```python
from build123d import *
from build123d import SkipClean  # not in build123d's __all__

# Parameters (mm, degrees)
F0_R        = 4.7625
F1_DEPTH    = 1.5875
F3_DEPTH    = 4.7625
F4_T1_DEPTH = 17.0592221242


# Not quite as in the source:
# - a fillet or chamfer that OpenCascade refuses, or shapes differently, is made with other operations: its cross-section is extruded or revolved along the edge and cut away or added


with BuildPart() as f1:
    # F0 (on Top) → F1 (new body)
    with BuildSketch(Plane.XY):
        with BuildLine():
            Line((-10.31875, 4.7625), (-10.31875, 0))
            ThreePointArc((-10.31875, 0), (0, -10.31875), (10.31875, 0))
            Line((10.31875, 0), (10.31875, 4.7625))
            ThreePointArc((10.31875, 4.7625), (0, 15.08125), (-10.31875, 4.7625))
        make_face()
        with Locations((0, -0.79375)):
            Circle(F0_R, mode=Mode.SUBTRACT)
    extrude(amount=F1_DEPTH)

    # F2 (on face) → F3 (join)
    with BuildSketch(Plane.XY.offset(1.5875)):
        with BuildLine():
            ThreePointArc((-4.7625, -0.79375), (0, 3.96875), (4.7625, -0.79375))
            Line((4.7625, -0.79375), (4.7625, 5.55625))
            ThreePointArc((4.7625, 5.55625), (0, 10.31875), (-4.7625, 5.55625))
            Line((-4.7625, 5.55625), (-4.7625, -0.79375))
        make_face()
    with SkipClean():  # cleaning this boolean's faces spoils the solid; the shape is the same uncleaned
        extrude(amount=F3_DEPTH)

    # F4: fillet of radius 1.27 on 2 edges, made by hand

    # F4_s2 → F4_t1 (cut)
    with BuildSketch(Plane.XY.offset(1.5875)):
        with BuildLine():
            ThreePointArc((4.7625, 4.1249388497), (4.075215964, 2.9965142376), (2.7572368421, 3.0894254076))
            ThreePointArc((2.7572368421, 3.0894254076), (4.2315922955, 1.3914348651), (4.7625, -0.79375))
            Line((4.7625, -0.79375), (4.7625, 4.1249388497))
        make_face()
        with BuildLine():
            ThreePointArc((-4.7625, 4.1249388497), (-4.075215964, 2.9965142376), (-2.7572368421, 3.0894254076))
            ThreePointArc((-2.7572368421, 3.0894254076), (-4.2315922955, 1.3914348651), (-4.7625, -0.79375))
            Line((-4.7625, -0.79375), (-4.7625, 4.1249388497))
        make_face()
    extrude(amount=F4_T1_DEPTH, mode=Mode.SUBTRACT)


solid = f1.part
```
Source: CAD feature listing. Evaluate the final solid. Frame: model axes, mm. A direction names the side the tool comes from. Give positions to 0.01 mm unless a question says otherwise; leave off trailing zeros. Loops run counter-clockwise (first coordinate to the right, second up) from the corner with the lowest first, then second, coordinate; pieces in that order, holes last. Notation, with made-up numbers: (29, 43) -> (44, 43) arc R22 ccw to (44, 68) -> close; hole circle Ø8 at (70.25, 78). An arc over 180 degrees is marked (long way). Put each result on its own line as item: value. Start each with the question number.
1) Cut plane A-A (x = 0). Return loops of the section in (y, z).
2) Contact query for flat-ended pins moving along their axis: P1, Ø1.5, axis at x = 4, z = 5.5, coming from the -Y side; P2, Ø0.7, axis at y = 5, z = 3, coming from the +X side. Output: stop coordinate, or through.
3) Reachability of faces 5 (the face through (0.105, 10.318, 3.935)), 6 (the face through (-4.762, 5, 4)), 7 (the face through (10.319, 2, 1)) from +Z, -Z, +X, -X, +Y, -Y: full face, straight path, thin tool, end or side. Return the list, or none.
4) Cut plane D-D (y = 7.25). Return loops of the section in (x, z), then the cut area to 3 significant figures.
5) Cut plane C-C (z = 1). Return loops of the section in (x, y) (1 decimal).
6) Material intervals for probe 1 along Y at (x, z) = (0, 1.2); probe 2 along Z at (x, y) = (4, 2.25); probe 3 along X at (y, z) = (5, 0.75), sorted ascending.
7) Draft query along X for faces 1 (the face through (0, 7, 6.35)), 2 (the face through (4.092, 3.006, 3.935)), 3 (the face through (-4.092, 3.006, 3.935)), 4 (the face through (4.762, 5, 4)). Return one class per face: released by +X, released by -X, zero draft, split by the parting line, or undercut.
8) Cut plane B-B (y = -3.5). Return loops of the section in (x, z).
Results are:
1. outline: (-10.32, 0) -> (-5.56, 0) -> (-5.56, 1.59) -> (-10.32, 1.59) -> close; (3.97, 0) -> (15.08, 0) -> (15.08, 1.59) -> (10.32, 1.59) -> (10.32, 6.35) -> (3.97, 6.35) -> close
2. P1: stops at y = 2.85
2. P2: stops at x = 4.76
3. face 5: +Z, +Y
3. face 6: +Z, -X, +Y, -Y
3. face 7: +Z, -Z, +X, +Y, -Y
4. outline: (-10.01, 0) -> (10.01, 0) -> (10.01, 1.59) -> (4.45, 1.59) -> (4.45, 6.35) -> (-4.45, 6.35) -> (-4.45, 1.59) -> (-10.01, 1.59) -> close
4. area: 74.2 mm2
5. outline: (-10.3, 0) arc R10.3 ccw to (10.3, 0) -> (10.3, 4.8) arc R10.3 ccw to (-10.3, 4.8) -> close; hole circle Ø9.5 at (0, -0.8)
6. probe 1: y = -10.32 to -5.56, 3.97 to 15.08
6. probe 2: z = 0 to 1.59
6. probe 3: x = -10.32 to 10.32
7. face 1: zero draft
7. face 2: undercut
7. face 3: undercut
7. face 4: released by +X
8. outline: (-9.71, 0) -> (-3.92, 0) -> (-3.92, 1.59) -> (-9.71, 1.59) -> close; (3.92, 0) -> (9.71, 0) -> (9.71, 1.59) -> (3.92, 1.59) -> close
